Work out the finished part from the listing and answer in its coordinate system (mm). Face numbers are marked on the shaded views. A direction names the side the tool comes from. Give positions to 0.01 mm unless a question says otherwise; leave off trailing zeros. Loops run counter-clockwise (first coordinate to the right, second up) from the corner with the lowest first, then second, coordinate; pieces in that order, holes last.
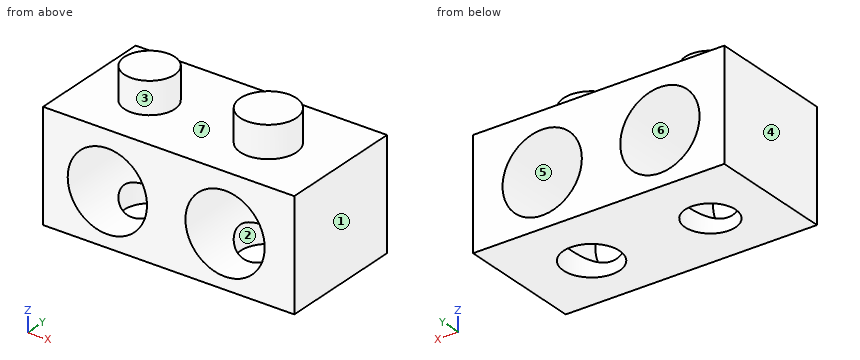
from build123d import *

# Parameters (mm, degrees)
F0_W      = 141.2794664502
F0_H      = 101.1280715466
F1_DEPTH  = 87.2775018215
F2_DEPTH  = 59.9578022957
F4_R      = 22.4182284803
F5_DEPTH  = 25.4
F3_R      = 20.138408071
F6_DEPTH  = 25.4
F7_DEPTH  = 164.3640697002
F8_DEPTH  = 163.5153144598
F9_DEPTH  = 63.5
F10_DEPTH = 63.5
F11_DEPTH = 25.4
F12_DEPTH = 25.4
F14_D     = 63.5
F17_D     = 63.5


with BuildPart() as f1:
    # F0 (on Top) → F1 (new body)
    with BuildSketch(Plane.XY):
        with Locations((-2.8060041368, 2.750582993)):
            Rectangle(F0_W, F0_H)
    extrude(amount=F1_DEPTH)

    # F2 (add): a face of the model
    f2_faces = [f1.faces().sort_by_distance(p)[0] for p in [
        (-73.4457373619, 2.750582993, 43.6387509108),
    ]]
    extrude(f2_faces, amount=F2_DEPTH)

    # F4 (on face) → F5 (join)
    with BuildSketch(Plane.XY.offset(87.2775018215)):
        with Locations((12.0112225413, 0)):
            Circle(F4_R)
    extrude(amount=F5_DEPTH)

    # F3 (on face) → F6 (join)
    with BuildSketch(Plane.XY.offset(87.2775018215)):
        with Locations((-83.1232145429, 0)):
            Circle(F3_R)
    extrude(amount=F6_DEPTH)

    # F7 (add): a face of the model
    f7_faces = [f1.faces().sort_by_distance(p)[0] for p in [
        (12.0112225413, 0, 112.6775018215),
    ]]
    extrude(f7_faces, amount=-F7_DEPTH)

    # F8 (add): a face of the model
    f8_faces = [f1.faces().sort_by_distance(p)[0] for p in [
        (-83.1232145429, 0, 112.6775018215),
    ]]
    extrude(f8_faces, amount=-F8_DEPTH)

    # F9 (cut): a face of the model
    f9_faces = [f1.faces().sort_by_distance(p)[0] for p in [
        (-83.1232145429, 0, -50.8378126383),
    ]]
    extrude(f9_faces, amount=-F9_DEPTH, mode=Mode.SUBTRACT)

    # F10 (cut): a face of the model
    f10_faces = [f1.faces().sort_by_distance(p)[0] for p in [
        (12.0112225413, 0, -51.6865678787),
    ]]
    extrude(f10_faces, amount=-F10_DEPTH, mode=Mode.SUBTRACT)

    # F11 (cut): a face of the model
    f11_faces = [f1.faces().sort_by_distance(p)[0] for p in [
        (-83.1232145429, 0, 12.6621873617),
    ]]
    extrude(f11_faces, amount=-F11_DEPTH, mode=Mode.SUBTRACT)

    # F12 (cut): a face of the model
    f12_faces = [f1.faces().sort_by_distance(p)[0] for p in [
        (12.0112225413, 0, 11.8134321213),
    ]]
    extrude(f12_faces, amount=-F12_DEPTH, mode=Mode.SUBTRACT)

    # F14 (through all)
    with Locations(Plane.XZ.offset(47.8134527802)):
        with Locations((12.4171413481, 41.448071599)):
            Hole(F14_D / 2)

    # F17 (through all)
    with Locations(Plane.XZ.offset(47.8134527802)):
        with Locations((-81.8664953113, 41.7736619711)):
            Hole(F17_D / 2)


solid = f1.part
Item 1: Flat-ended cylindrical pins translate along their axes: pin 1 Ø4 at (x, y) = (22.5, -23) entering from +Z; pin 2 Ø12 at (x, y) = (-77, 2.5) entering from -Z; pin 3 Ø10 at (x, z) = (-95, 92.5) entering from +Y; pin 4 Ø6 at (x, z) = (6, 70) entering from +Y. Find the tip coordinate at first contact, or state that the pin passes through.
Item 2: Find section C-C, the plane y = -13. Write down the section's boundary in (x, z).
Item 3: Find section A-A, the plane x = -4. Write down the section's boundary in (y, z).
Item 4: For the marked faces 1, 2 and 3, determine the directions among +Z, -Z, +X, -X, +Y, -Y from which every point of the face is accessible in a straight line to the end or side of a thin tool.
Item 5: Determine the mould class of the marked faces 4, 5, 6 and 7 for opening direction Z: released by +Z, released by -Z, zero draft, split by the parting line, or undercut.
Item 6: Find section B-B, the plane z = 24. Write down the section's boundary in (x, y), plus the area to 3 significant figures.
Item 7: Find section D-D, the plane x = -54. Write down the section's boundary in (y, z).
Item 8: Consider line 1 (X direction, y = 16, z = 41); line 2 (X direction, y = 18.5, z = 37.5); line 3 (Z direction, x = -23.5, y = 42.5). Determine where each line is inside the solid, lowest interval first.
Ans:
1. pin 1: stops at z = 87.28
1. pin 2: stops at z = 71.61
1. pin 3: stops at y = 18.93
1. pin 4: stops at y = 53.31
2. outline: (-133.4, 0) - (-98.5, 0) - (-98.5, 14.73) arc R31.75 cw (long way) to (-67.74, 13.34) - (-67.74, 0) - (-6.25, 0) - (-6.25, 15.77) arc R31.75 cw (long way) to (30.28, 15.2) - (30.28, 0) - (67.83, 0) - (67.83, 87.28) - (30.28, 87.28) - (30.28, 112.68) - (-6.25, 112.68) - (-6.25, 87.28) - (-67.74, 87.28) - (-67.74, 112.68) - (-98.5, 112.68) - (-98.5, 87.28) - (-133.4, 87.28) - close
3. outline: (-47.81, 0) - (-15.69, 0) - (-15.69, 14.27) - (-47.81, 14.27) - close; (-47.81, 68.62) - (53.31, 68.62) - (53.31, 87.28) - (15.69, 87.28) - (15.69, 112.68) - (-15.69, 112.68) - (-15.69, 87.28) - (-47.81, 87.28) - close; (15.69, 0) - (53.31, 0) - (53.31, 14.27) - (15.69, 14.27) - close
4. face 1: +Z, -Z, +X, +Y, -Y
4. face 2: -Z
4. face 3: +Z
5. face 4: zero draft
5. face 5: undercut
5. face 6: undercut
5. face 7: released by +Z
6. outline: (-133.4, -47.81) - (-108.18, -47.81) - (-108.18, 53.31) - (-133.4, 53.31) - close; (-55.56, -47.81) - (-14.11, -47.81) - (-14.11, 53.31) - (-55.56, 53.31) - close; (38.94, -47.81) - (67.83, -47.81) - (67.83, 53.31) - (38.94, 53.31) - close
6. area: 9,660 mm2
7. outline: (-47.81, 0) - (53.31, 0) - (53.31, 26.56) - (-47.81, 26.56) - close; (-47.81, 56.99) - (53.31, 56.99) - (53.31, 87.28) - (-47.81, 87.28) - close
8. line 1: x = -133.4 to -113.61, -50.13 to -19.33, 44.16 to 67.83
8. line 2: x = -133.4 to -113.33, -50.41 to -19.09, 43.92 to 67.83
8. line 3: z = 0 to 87.28
